Autodesk Inventor part; units mm, degrees
ref_plane "YZ Plane" through (0, 0, 0) normal (1, 0, 0) x (0, 1, 0)
ref_plane "XZ Plane" through (0, 0, 0) normal (0, 1, 0) x (-1, 0, 0)
ref_plane "XY Plane" through (0, 0, 0) normal (0, 0, 1) x (1, 0, 0)
sketch "Sketch1" plane through (0, 0, 0) normal (0, 1, 0) x (-1, 0, 0)
  circle A0 centre (0, 0) radius 3.5
  circle A1 centre (0, 0) radius 2
  dimension "d0" = 7
  dimension "d2" = 4
extrude "Extrusion1" add sketch "Sketch1" against normal blind 3
extrude "Extrusion2" add sketch "Sketch1" along normal blind 0.5 contours A0 | A1
sketch "Sketch2" plane through (0, 0.5, 0) normal (0, 1, 0) x (1, 0, 0)
  circle A0 centre (0, 0) radius 2.5
  circle A1 centre (0, 0) radius 1.5
  dimension "d10" = 5
  dimension "d11" = 3
extrude "Extrusion4" add sketch "Sketch2" along normal blind 3.25
fillet "Fillet1" radius 0.4 2 edges at (-2.5, 0.5, 0) (2, 0, 0)
extrude "Extrusion5" cut sketch "Sketch2" against normal blind 3.25 contours A1
properties part number "m.2 support"
Design review of the part built by this model. Coordinates are the model's own, in mm. A direction names the side the tool comes from. Round coordinates to 2 decimals unless told otherwise and drop trailing zeros. Write each loop counter-clockwise with the first axis right and the second up, starting at its lowest first coordinate (ties: lowest second). Pieces come first, ordered by that corner, then holes. Notation, with made-up numbers: (-3, 82) - (23, 82) arc R24 cw to (23, 95) - close; hole circle Ø7 at (73, 82.5). An arc over 180 degrees is marked (long way). Use a Markdown table: item, result. Add a question column.
1. We need section A-A (x = 0). State the section outline as (y, z) points.
2. Mouldability with a two-part tool opening along Z and no side actions: class faces 3 (the face through (-2, -3, -2)), 4 (the face through (0, -2, -2)), 5 (the face through (-3.233, -1.226, -1.341)) as +Z half, -Z half, draft (parallel to the pull), parting line (faces both ways), or undercut.
3. We need section D-D (y = -0.5). State the section outline as (x, z) points, then the cut area to 3 significant figures.
4. We need section B-B (z = 0). State the section outline as (x, y) points, then the cut area to 3 significant figures.
5. Wall thickness on probe 1 along X at (y, z) = (1.9, 0); probe 2 along Z at (x, y) = (0, -1.25): over which ranges is each line inside the solid? List them lowest first.
6. For faces 1 (the face through (-1.5, 1.85, 0.07)), 2 (the face through (1, 0.5, 3)), list the 3-axis set-ups (+Z, -Z, +X, -X, +Y, -Y) from which the entire face can be reached by the end or side of a thin tool; tool diameter is ignored.
7. We need section C-C (y = 1.5). State the section outline as (x, z) points, then the cut area to 3 significant figures.
Output:
| question | item | result |
|---|---|---|
| 1 | outline | (-3, -3.5) - (0.5, -3.5) - (0.5, -2.9) arc R0.4 cw to (0.9, -2.5) - (3.75, -2.5) - (3.75, -1.5) - (0, -1.5) - (0, -1.6) arc R0.4 cw to (-0.4, -2) - (-3, -2) - close; (-3, 2) - (-0.4, 2) arc R0.4 cw to (0, 1.6) - (0, 1.5) - (3.75, 1.5) - (3.75, 2.5) - (0.9, 2.5) arc R0.4 cw to (0.5, 2.9) - (0.5, 3.5) - (-3, 3.5) - close |
| 2 | face 3 | draft |
| 2 | face 4 | undercut |
| 2 | face 5 | parting line |
| 3 | outline | circle Ø7 at (0, 0); hole circle Ø4 at (0, 0) |
| 3 | area | 25.9 mm2 |
| 4 | outline | (-3.5, -3) - (-2, -3) - (-2, -0.4) arc R0.4 cw to (-1.6, 0) - (-1.5, 0) - (-1.5, 3.75) - (-2.5, 3.75) - (-2.5, 0.9) arc R0.4 cw to (-2.9, 0.5) - (-3.5, 0.5) - close; (1.5, 0) - (1.6, 0) arc R0.4 cw to (2, -0.4) - (2, -3) - (3.5, -3) - (3.5, 0.5) - (2.9, 0.5) arc R0.4 cw to (2.5, 0.9) - (2.5, 3.75) - (1.5, 3.75) - close |
| 4 | area | 17.6 mm2 |
| 5 | probe 1 | x = -2.5 to -1.5, 1.5 to 2.5 |
| 5 | probe 2 | z = -3.5 to -2, 2 to 3.5 |
| 6 | face 1 | +Y, -Y |
| 6 | face 2 | +Y |
| 7 | outline | circle Ø5 at (0, 0); hole circle Ø3 at (0, 0) |
| 7 | area | 12.6 mm2 |
